```python
from build123d import *

# Parameters (mm, degrees)
FILLET2_R     = 0.344
CHAMFER2_SIZE = 0.2


with BuildPart() as part:
    # Sketch1 → Revolve1 (revolve)
    with BuildSketch(Plane.XY, mode=Mode.PRIVATE) as revolve1_sk:
        Polygon((10.5, 0), (10.5, 4), (9.5, 4), (9.5, 3.9), (9.3, 3.9), (9.3, 4), (8.7, 4), (8.7, 3.9), (8.5, 3.9), (8.5, 4), (7.5, 4), (7.5, 0), (8.5, 0), (8.5, 0.1), (8.7, 0.1), (8.7, 0), (9.3, 0), (9.3, 0.1), (9.5, 0.1), (9.5, 0), align=None)
    revolve(revolve1_sk.sketch.rotate(Axis((0, 2, 0), (0, -1, 0)), 90), axis=Axis((0, 2, 0), (0, -1, 0)))

    # Fillet2
    fillet2_edges = [part.edges().sort_by_distance(p)[0] for p in [
        (0, 0, -10.5),
        (0, 4, -10.5),
    ]]
    fillet(fillet2_edges, radius=FILLET2_R)

    # Chamfer2
    chamfer2_edges = [part.edges().sort_by_distance(p)[0] for p in [
        (0, 4, -7.5),
        (0, 0, -7.5),
    ]]
    chamfer(chamfer2_edges, length=CHAMFER2_SIZE)


solid = part.part
```
Input: part model. Units: mm. Frame: model coordinates. Round coordinates to 2 decimals unless told otherwise and drop trailing zeros. Loops run counter-clockwise (first coordinate to the right, second up) from the corner with the lowest first, then second, coordinate; pieces in that order, holes last. Notation, with made-up numbers: (-20, -19.5) -> (12, -19.5) arc R30 ccw to (12, 2.5) -> close; hole circle Ø3 at (-3.75, -32). An arc over 180 degrees is marked (long way). Use one line per item in the form item = value. Start each with the question number.
Item 1: Section query A-A on y = 2.8. Return the cut outline in (x, z), then the cut area to 3 significant figures.
Item 2: Contact query for a flat-ended pin moving along its axis: pin 1 Ø1 at (x, y) = (3.5, 0.5) entering from +Z. Output: stop coordinate, or through.
Item 3: Material intervals for L1, parallel to Z at x = 4.75, y = 2.75; L2, parallel to X at y = 0.25, z = -6.75; L3, parallel to Z at x = 9.75, y = 1.65, sorted ascending. Write a range as from..to.
Ans:
q1.outline = circle Ø21 at (0, 0); hole circle Ø15 at (0, 0)
q1.area = 170 mm^2
q2.pin_1 = 10.06
q3.L1 = -9.36..-5.8, 5.8..9.36
q3.L2 = -8.03..-3.27, 3.27..8.03
q3.L3 = -3.9..3.9
